Here's the drawing with two shaded views (mm, measured from the low corner). I have some questions. A direction names the side the tool comes from. Coordinates: 2 decimals unless noted, no trailing zeros. Loops run counter-clockwise (first coordinate to the right, second up) from the corner with the lowest first, then second, coordinate; pieces in that order, holes last. Notation, with made-up numbers: (69, -5) -> (126, -5) arc R21 ccw to (126, 16) -> close; hole circle Ø5 at (0.25, 15). An arc over 180 degrees is marked (long way). Answer as a JSON object with one key per item and string values. Group by question number.
1) Which directions (+Z, -Z, +X, -X, +Y, -Y) give clear straight access to the entire face, cutting with the end or side of a thin tool? Please do the marked faces 1 and 2.
2) I want a section at C-C (x = 43). Write out the boundary of the cut face in (y, z).
3) I'm going to push flat-ended pins straight in: pin 1 (0.8 mm diameter, centred on x = 52, z = 14, fed in from +Y); pin 2 (2 mm diameter, centred on y = 31, z = 9, fed in from +X); pin 3 (7 mm diameter, centred on y = 36, z = 10.5, fed in from -X); pin 4 (0.8 mm diameter, centred on x = 80, z = 14, fed in from +Y). Where does each tip first touch, or does it pass through?
4) I want a section at B-B (y = 3). Write out the boundary of the cut face in (x, z).
5) I want a section at A-A (x = 80). Write out the boundary of the cut face in (y, z).
6) I need wall thicknesses on probe 1 along Y at (x, z) = (80, 14.05); probe 2 along Y at (x, z) = (46, 14.1); probe 3 along Z at (x, y) = (32, 3). Which ranges of each line are inside material? Lowest first, please. Write a range as [from, to].
7) I want a section at D-D (y = 22). Write out the boundary of the cut face in (x, z), then the cut area to 3 significant figures.
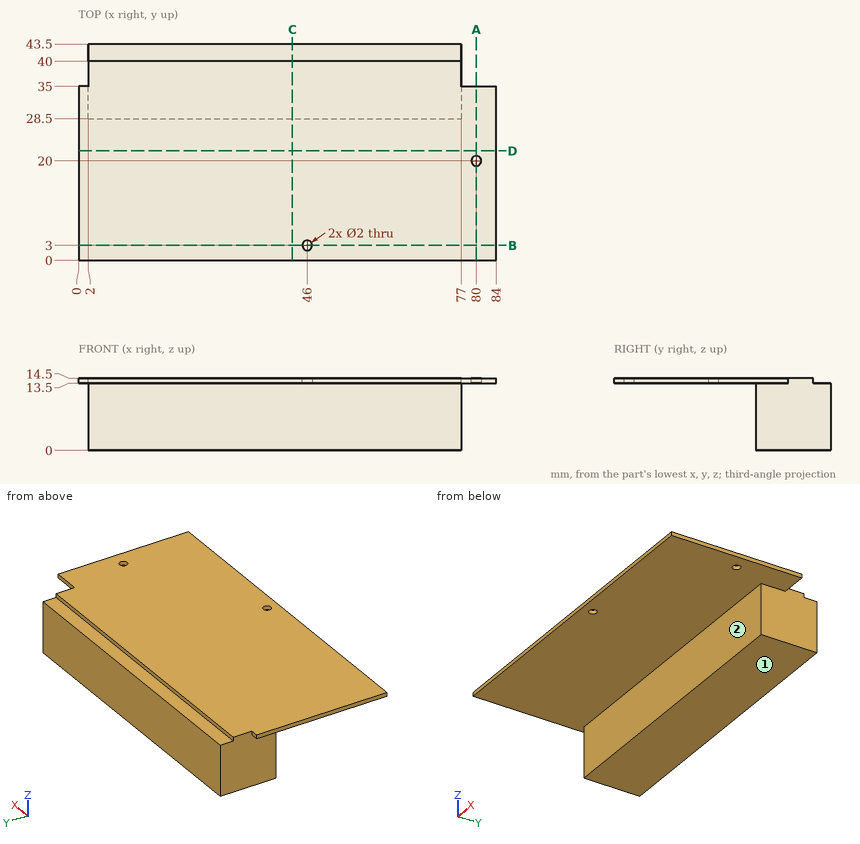
Determined:
{
 "1": {"face 1": "-Z, +X, -X, +Y, -Y", "face 2": "-Z, +X, -X, -Y"},
 "2": {"outline": "(0, 13.5) -> (28.5, 13.5) -> (28.5, 0) -> (43.5, 0) -> (43.5, 13.5) -> (40, 13.5) -> (40, 14.5) -> (0, 14.5) -> close"},
 "3": {"pin 1": "y = 40", "pin 2": "x = 77", "pin 3": "x = 0", "pin 4": "y = 35"},
 "4": {"outline": "(0, 13.5) -> (45, 13.5) -> (45, 14.5) -> (0, 14.5) -> close; (47, 13.5) -> (84, 13.5) -> (84, 14.5) -> (47, 14.5) -> close"},
 "5": {"outline": "(0, 13.5) -> (19, 13.5) -> (19, 14.5) -> (0, 14.5) -> close; (21, 13.5) -> (35, 13.5) -> (35, 14.5) -> (21, 14.5) -> close"},
 "6": {"probe 1": "[0, 19], [21, 35]", "probe 2": "[0, 2], [4, 40]", "probe 3": "[13.5, 14.5]"},
 "7": {"outline": "(0, 13.5) -> (84, 13.5) -> (84, 14.5) -> (0, 14.5) -> close", "area": "84.0 mm^2"}
}
